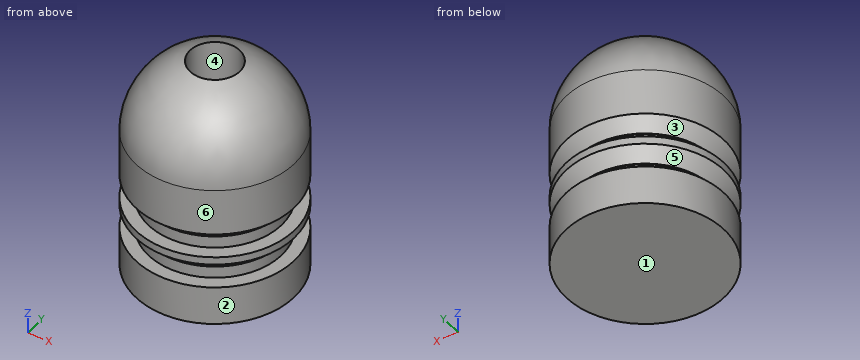
from build123d import *

# Parameters (mm, degrees)
F0_R      = 20.25
F1_DEPTH  = 10
F2_R      = 17
F3_DEPTH  = 3.25
F4_R      = 20.25
F4_R_2    = 17
F5_DEPTH  = 5
F6_R      = 17
F7_DEPTH  = 3.25
F8_R      = 20.25
F8_R_2    = 17
F9_DEPTH  = 25
F10_DEPTH = 5
F11_DEPTH = 5
F13_R     = 6.35
F13_R_2   = 0.25
F14_DEPTH = 20
F15_SIZE  = 3


# Not quite as in the source:
# - a fillet or chamfer that OpenCascade refuses, or shapes differently, is made with other operations: its cross-section is extruded or revolved along the edge and cut away or added


with BuildPart() as f1:
    # F0 (on Top) → F1 (new body)
    with BuildSketch(Plane.XY):
        Circle(F0_R)
    extrude(amount=F1_DEPTH)

    # F2 (on face) → F3 (join)
    with BuildSketch(Plane.XY.offset(10)):
        Circle(F2_R)
    extrude(amount=F3_DEPTH)

    # F4 (on face) → F5 (join)
    with BuildSketch(Plane.XY.offset(13.25)):
        Circle(F4_R)
        Circle(F4_R_2, mode=Mode.SUBTRACT)
        Circle(F4_R_2)
    extrude(amount=F5_DEPTH)

    # F6 (on face) → F7 (join)
    with BuildSketch(Plane.XY.offset(18.25)):
        Circle(F6_R)
    extrude(amount=F7_DEPTH)

    # F8 (on face) → F9 (join)
    with BuildSketch(Plane.XY.offset(21.5)):
        Circle(F8_R)
        Circle(F8_R_2, mode=Mode.SUBTRACT)
        Circle(F8_R_2)
    extrude(amount=F9_DEPTH)

    # F10 (add): a face of the model
    f10_faces = [f1.faces().sort_by_distance(p)[0] for p in [
        (0, 0, 46.5),
    ]]
    extrude(f10_faces, amount=F10_DEPTH)

    # F11 (add): a face of the model
    f11_faces = [f1.faces().sort_by_distance(p)[0] for p in [
        (0, 0, 51.5),
    ]]
    extrude(f11_faces, amount=F11_DEPTH)

    # F12: fillet of radius 20 on 1 edges, made by hand

    # F12_s1 → F12_t2 (revolve, cut)
    with BuildSketch(Plane.XZ):
        with BuildLine():
            add(Edge.make_bspline(
                [(20.25, 36.5), (20.25, 56.5), (0.25, 56.5)],
                knots=[0, 0, 0, 1, 1, 1], degree=2, weights=[1, 0.6666666667, 1]))
            Line((0.25, 56.5), (20.25, 56.5))
            Line((20.25, 56.5), (20.25, 36.5))
        make_face()
    revolve(axis=Axis((0, 0, 56.5), (0, 0, 1)), mode=Mode.SUBTRACT)

    # F13 (on face) → F14 (cut)
    with BuildSketch(Plane.XY.offset(56.5)):
        Circle(F13_R)
        Circle(F13_R_2, mode=Mode.SUBTRACT)
        Circle(F13_R_2)
    extrude(amount=-F14_DEPTH, mode=Mode.SUBTRACT)

    # F15
    f15_edges = [f1.edges().sort_by_distance(p)[0] for p in [
        (-20.25, 0, 13.25),
        (-20.25, 0, 21.5),
    ]]
    chamfer(f15_edges, length=F15_SIZE)


solid = f1.part
The model under review builds one solid part; all positions refer to its coordinate system, in mm. Face numbers are marked on the shaded views. A direction names the side the tool comes from. Coordinates: 2 decimals unless noted, no trailing zeros. Write each loop counter-clockwise with the first axis right and the second up, starting at its lowest first coordinate (ties: lowest second). Pieces come first, ordered by that corner, then holes. Notation, with made-up numbers: (71, 28) -> (118, 28) arc R14 cw to (118, 50) -> close; hole circle Ø2 at (-6.5, 8.25). An arc over 180 degrees is marked (long way). Answer in a Markdown table with one row per item.
1. Wall thickness on probe 1 along Z at (x, y) = (0.5, 1); probe 2 along X at (y, z) = (0, 47); probe 3 along Y at (x, z) = (0, 48): over which ranges is each line inside the solid? List them lowest first. Write a range as [from, to].
Answers below:
| item | result |
|---|---|
| probe 1 | z = [0, 36.5] |
| probe 2 | x = [-17.07, -6.35], [6.35, 17.07] |
| probe 3 | y = [-16.39, -6.35], [6.35, 16.39] |
2. For the marked faces 4, 5 and 6, list the 3-axis set-ups (+Z, -Z, +X, -X, +Y, -Y) from which the entire face can be reached by the end or side of a thin tool; tool diameter is ignored.
Answers below:
| item | result |
|---|---|
| face 4 | +Z |
| face 5 | none |
| face 6 | +Z, -Z |
3. Clearance check with flat-ended pins moving along their axes: pin 1 Ø5 at (y, z) = (12.5, 37) entering from -X; pin 2 Ø10 at (x, y) = (-5.5, 10) entering from -Z; pin 3 Ø6 at (x, y) = (-9.5, -14.5) entering from +Z; pin 4 Ø12 at (y, z) = (4.5, 49) entering from -X. State where each tip first meets the part, or that it passes through.
Answers below:
| item | result |
|---|---|
| pin 1 | stops at x = -17.6 |
| pin 2 | stops at z = 0 |
| pin 3 | stops at z = 50.41 |
| pin 4 | stops at x = -18.78 |
4. Draft analysis for pull direction Z (two halves, no side actions). For the marked faces 1, 2 and 3, state which applies: +Z half, -Z half, draft (parallel to the pull), parting line (faces both ways), or undercut.
Answers below:
| item | result |
|---|---|
| face 1 | -Z half |
| face 2 | draft |
| face 3 | undercut |
5. We need section A-A, the plane z = 20.5. State the section outline as (x, y) points.
Answers below:
| item | result |
|---|---|
| outline | circle Ø34 at (0, 0) |
